Autodesk Inventor part; units mm, degrees
ref_plane "YZ Plane" through (0, 0, 0) normal (1, 0, 0) x (0, 1, 0)
ref_plane "XZ Plane" through (0, 0, 0) normal (0, 1, 0) x (-1, 0, 0)
ref_plane "XY Plane" through (0, 0, 0) normal (0, 0, 1) x (1, 0, 0)
sketch "Sketch1" plane through (0, 0, 0) normal (0, 0, 1) x (1, 0, 0)
  line L0 (0, 0) -> (182, 0)
  line L1 (182, 0) -> (182, 52)
  line L2 (182, 52) -> (0, 52)
  line L3 (0, 52) -> (0, 0)
  dimension "d0" = 182
  dimension "d1" = 52
extrude "Extrusion1" add sketch "Sketch1" along normal blind 50
sketch "Sketch2" plane through (182, 0, 0) normal (1, 0, 0) x (0, 0, -1)
  line L0 (0, 52) -> (-50, 52)
  line L1 (-25, 52) -> (-50, 26)
  line L2 (-50, 0) -> (-50, 52)
  line L3 (-25, 52) -> (-50, 52)
  line L4 (-50, 52) -> (-50, 26)
  point P0 (0, 0)
extrude "Extrusion2" cut sketch "Sketch2" against normal through all
sketch "Sketch3" plane through (0, 0, 0) normal (0, -1, 0) x (1, 0, 0)
  line L0 (0, 50) -> (182, 50)
  line L1 (182, 0) -> (0, 0)
  line L2 (0, 0) -> (0, 50)
  line L3 (0, 50) -> (182, 50)
  line L4 (182, 50) -> (182, 0)
  line L5 (-6, -6) -> (188, -6)
  line L6 (188, -6) -> (188, 52)
  line L7 (-6, 52) -> (-6, -6)
  line L8 (182, 50) -> (0, 50)
  line L9 (188, 52) -> (-6, 52)
  dimension "d6" = 6
extrude "Extrusion3" add sketch "Sketch3" against normal blind 4 contours L0 L4 L1 L2 | L7 L9 L6 L5
fillet "Fillet1" radius 2 4 edges at (188, 2, -6) (188, 2, 52) (-6, 2, 52) (-6, 2, -6)
properties part number "Early-944_Radio_Plug"
Geometry check sheet. Reference: the model listing, model coordinates, mm. A direction names the side the tool comes from. Give positions to 0.01 mm unless a question says otherwise; leave off trailing zeros. Write each loop counter-clockwise with the first axis right and the second up, starting at its lowest first coordinate (ties: lowest second). Pieces come first, ordered by that corner, then holes. Notation, with made-up numbers: (85.25, 75.5) - (103.25, 75.5) arc R15 ccw to (103.25, 91.5) - close; hole circle Ø3 at (65.5, -12.5). An arc over 180 degrees is marked (long way). Use a Markdown table: item, result.
Q1. Thickness scan on L1, parallel to X at y = 31, z = 33; L2, parallel to Z at x = 94.5, y = 26; L3, parallel to Y at x = 114, z = 34.5. Record the ranges inside material, lowest first. Write a range as [from, to].
Computed:
| item | result |
|---|---|
| L1 | x = [0, 182] |
| L2 | z = [0, 50] |
| L3 | y = [0, 42.12] |
Q2. Section check B-B, the plane x = 106. Enter the section's corners in (y, z), then the cut area to 3 significant figures.
Computed:
| item | result |
|---|---|
| outline | (0, -6) - (4, -6) - (4, 0) - (52, 0) - (52, 25) - (26, 50) - (4, 50) - (4, 52) - (0, 52) - close |
| area | 2,310 mm² |
Q3. Set-up check for faces 4 (the face through (90, 15, 50)), 5 (the face through (90, 28, 0)), 6 (the face through (0, 28, 25)): record each of +Z, -Z, +X, -X, +Y, -Y from which the full face is reachable in a straight line by a thin tool's end or side.
Computed:
| item | result |
|---|---|
| face 4 | +Z, +X, -X, +Y |
| face 5 | -Z, +X, -X, +Y |
| face 6 | +Z, -Z, -X, +Y |
Q4. Section check D-D, the plane z = 23. Enter the section's corners in (x, y).
Computed:
| item | result |
|---|---|
| outline | (-6, 0) - (188, 0) - (188, 4) - (182, 4) - (182, 52) - (0, 52) - (0, 4) - (-6, 4) - close |
Q5. Go/stop test with flat-tipped pins: P1, Ø24, axis at y = 31, z = 12.5, coming from the +X side; P2, Ø2, axis at x = 92.5, y = 22, coming from the -Z side; P3, Ø1, axis at y = 34.5, z = 24.5, coming from the -X side; P4, Ø5, axis at x = 52, z = 34.5, coming from the -Y side. Record where each tip stops, or that it passes through.
Computed:
| item | result |
|---|---|
| P1 | stops at x = 182 |
| P2 | stops at z = 0 |
| P3 | stops at x = 0 |
| P4 | stops at y = 0 |
Q6. Section check C-C, the plane y = 21.5. Enter the section's corners in (x, z), then the cut area to 3 significant figures.
Computed:
| item | result |
|---|---|
| outline | (0, 0) - (182, 0) - (182, 50) - (0, 50) - close |
| area | 9,100 mm² |
Q7. Section check A-A, the plane z = 34. Enter the section's corners in (x, y).
Computed:
| item | result |
|---|---|
| outline | (-6, 0) - (188, 0) - (188, 4) - (182, 4) - (182, 42.64) - (0, 42.64) - (0, 4) - (-6, 4) - close |
Q8. Draft check along Z on faces 1 (the face through (188, 2, 23)), 2 (the face through (90, 2, -6)), 3 (the face through (92.274, 39.182, 37.325)). Enter one of: pulls with the +Z half, pulls with the -Z half, needs draft (parallel to the pull), parting line crosses it, or undercut.
Computed:
| item | result |
|---|---|
| face 1 | needs draft |
| face 2 | pulls with the -Z half |
| face 3 | pulls with the +Z half |
